from build123d import *

# Parameters (mm, degrees)
EXTRUDE_1_DEPTH     = 51.5
FILLET_2_R          = 6
SKETCH_2_W          = 41
SKETCH_2_H          = 41
CUT_EXTRUDE_1_DEPTH = 48.5
SKETCH_3_W          = 36
SKETCH_3_H          = 45.5
CUT_EXTRUDE_2_DEPTH = 54
SKETCH_4_W          = 36
SKETCH_4_H          = 45.5
CUT_EXTRUDE_3_DEPTH = 54
CUT_EXTRUDE_4_DEPTH = 6.5
CUT_EXTRUDE_5_DEPTH = 4


with BuildPart() as part:
    # 草图1 → 凸台-拉伸1 (new body)
    with BuildSketch(Plane(origin=(0, 0, 0), x_dir=(1, 0, 0), z_dir=(0, 1, 0))):
        with BuildLine():
            Line((-18, -24), (18, -24))
            ThreePointArc((18, -24), (22.242640687, -22.242640687), (24, -18))
            Line((24, -18), (24, 18))
            ThreePointArc((24, 18), (22.242640687, 22.242640687), (18, 24))
            Line((18, 24), (-18, 24))
            ThreePointArc((-18, 24), (-22.242640687, 22.242640687), (-24, 18))
            Line((-24, 18), (-24, -18))
            ThreePointArc((-24, -18), (-22.242640687, -22.242640687), (-18, -24))
        make_face()
    extrude(amount=EXTRUDE_1_DEPTH)

    # 圆角2
    fillet_2_edges = [part.edges().sort_by_distance(p)[0] for p in [
        (22.242640687, 51.5, -22.242640687),
        (24, 51.5, 0),
        (22.242640687, 51.5, 22.242640687),
        (0, 51.5, 24),
        (-22.242640687, 51.5, 22.242640687),
        (-24, 51.5, 0),
        (-22.242640687, 51.5, -22.242640687),
        (0, 51.5, -24),
    ]]
    fillet(fillet_2_edges, radius=FILLET_2_R)

    # 草图2 → 切除-拉伸1 (cut)
    with BuildSketch(Plane.XZ):
        Rectangle(SKETCH_2_W, SKETCH_2_H)
    extrude(amount=-CUT_EXTRUDE_1_DEPTH, mode=Mode.SUBTRACT)

    # 草图3 → 切除-拉伸2 (cut)
    with BuildSketch(Plane(origin=(0, 0, -24), x_dir=(-1, 0, 0), z_dir=(0, 0, -1))):
        with Locations((0, 22.75)):
            Rectangle(SKETCH_3_W, SKETCH_3_H)
    extrude(amount=-CUT_EXTRUDE_2_DEPTH, mode=Mode.SUBTRACT)

    # 草图4 → 切除-拉伸3 (cut)
    with BuildSketch(Plane.ZY.offset(24)):
        with Locations((0, 22.75)):
            Rectangle(SKETCH_4_W, SKETCH_4_H)
    extrude(amount=-CUT_EXTRUDE_3_DEPTH, mode=Mode.SUBTRACT)

    # 草图5 → 切除-拉伸4 (cut)
    with BuildSketch(Plane.XZ):
        with BuildLine():
            Line((-17.5, -23), (17.5, -23))
            ThreePointArc((17.5, -23), (21.389087297, -21.389087297), (23, -17.5))
            Line((23, -17.5), (23, 17.5))
            ThreePointArc((23, 17.5), (21.389087297, 21.389087297), (17.5, 23))
            Line((17.5, 23), (-17.5, 23))
            ThreePointArc((-17.5, 23), (-21.389087297, 21.389087297), (-23, 17.5))
            Line((-23, 17.5), (-23, -17.5))
            ThreePointArc((-23, -17.5), (-21.389087297, -21.389087297), (-17.5, -23))
        make_face()
    extrude(amount=-CUT_EXTRUDE_4_DEPTH, mode=Mode.SUBTRACT)

    # 草图8 → 切除-拉伸5 (cut)
    with BuildSketch(Plane.XZ):
        with BuildLine():
            Line((18, -22.977225575), (18, -24))
            ThreePointArc((18, -24), (22.242640687, -22.242640687), (24, -18))
            Line((24, -18), (22.977225575, -18))
            ThreePointArc((22.977225575, -18), (21.389087297, -21.389087297), (18, -22.977225575))
        make_face()
        with BuildLine():
            Line((22.977225575, 18), (24, 18))
            ThreePointArc((24, 18), (22.242640687, 22.242640687), (18, 24))
            Line((18, 24), (18, 22.977225575))
            ThreePointArc((18, 22.977225575), (21.389087297, 21.389087297), (22.977225575, 18))
        make_face()
        with BuildLine():
            Line((-18, 22.977225575), (-18, 24))
            ThreePointArc((-18, 24), (-22.242640687, 22.242640687), (-24, 18))
            Line((-24, 18), (-22.977225575, 18))
            ThreePointArc((-22.977225575, 18), (-21.389087297, 21.389087297), (-18, 22.977225575))
        make_face()
        with BuildLine():
            Line((-22.977225575, -18), (-24, -18))
            ThreePointArc((-24, -18), (-22.242640687, -22.242640687), (-18, -24))
            Line((-18, -24), (-18, -22.977225575))
            ThreePointArc((-18, -22.977225575), (-21.389087297, -21.389087297), (-22.977225575, -18))
        make_face()
    extrude(amount=-CUT_EXTRUDE_5_DEPTH, mode=Mode.SUBTRACT)


solid = part.part
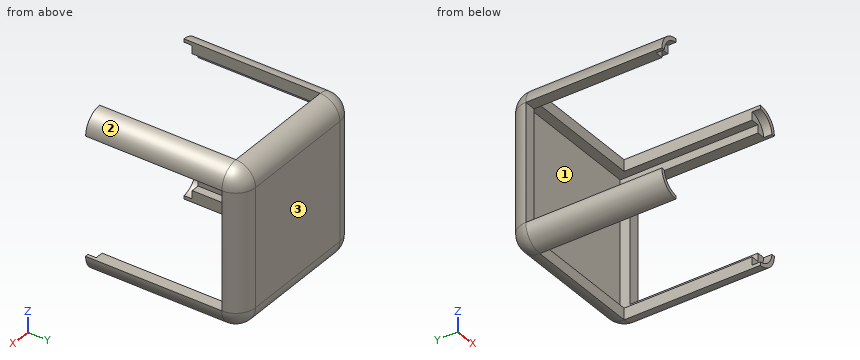
The listing builds one solid part. Answer for the finished solid, in the listing's coordinates (mm). Face numbers are marked on the shaded views. Give positions to 0.01 mm unless a question says otherwise; leave off trailing zeros. Loops run counter-clockwise (first coordinate to the right, second up) from the corner with the lowest first, then second, coordinate; pieces in that order, holes last. Notation, with made-up numbers: (32.25, 78.5) - (64.25, 78.5) arc R21 ccw to (64.25, 87.5) - close; hole circle Ø5 at (-40, 77.5). An arc over 180 degrees is marked (long way). Use one line per item in the form item = value.
1. Section D-D on x = -19 is taken. Give the vertices of the cut face in (y, z), then the cut area to 3 significant figures.
Calculated:
outline = (4, -23.92) - (45.5, -23.92) arc R5.92 ccw to (51.42, -18) - (51.42, 18) arc R5.92 ccw to (45.5, 23.92) - (4, 23.92) - (4, 22.79) - (6.5, 22.79) - (6.5, 20.5) - (48.5, 20.5) - (48.5, -20.5) - (6.5, -20.5) - (6.5, -22.79) - (4, -22.79) - close
area = 417 mm^2
2. Section B-B on x = 1 is taken. Give the vertices of the cut face in (y, z), then the cut area to 3 significant figures.
Calculated:
outline = (45.5, -24) arc R6 ccw to (51.5, -18) - (51.5, 18) arc R6 ccw to (45.5, 24) - (45.5, 20.5) - (48.5, 20.5) - (48.5, -20.5) - (45.5, -20.5) - close
area = 150 mm^2
3. Find the intervals of material crossed by line 1 along Y through (x, z) = (-7.5, 15); line 2 along X through (y, z) = (20.5, 19.5); line 3 along X through (y, z) = (42, -21.5), in increasing order. Write a range as [from, to].
Calculated:
line_1 = [48.5, 51.5]
line_2 = [-23.81, -20.5], [20.5, 23.81]
line_3 = [-22.87, -18], [18, 22.87]
4. Given pin 1 Ø4 at (x, y) = (-22, 25) entering from +Z; pin 2 Ø10 at (x, z) = (-3, 11.5) entering from -Y; pin 3 Ø3 at (x, z) = (21.5, 3.5) entering from -Y; pin 4 Ø20.5 at (y, z) = (34, 8) entering from +X, each flat-ended and moving along its own axis, determine where each tip first touches the part or whether it passes through.
Calculated:
pin_1 = 23.66
pin_2 = 48.5
pin_3 = 45.5
pin_4 = 24
5. Section A-A on y = 32.5 is taken. Give the vertices of the cut face in (x, z), then the cut area to 3 significant figures.
Calculated:
outline = (-24, -18) arc R6 ccw to (-18, -24) - (-18, -20.5) - (-20.5, -20.5) - (-20.5, -18) - close; (-24, 18) - (-20.5, 18) - (-20.5, 20.5) - (-18, 20.5) - (-18, 24) arc R6 ccw to start; (18, -24) arc R6 ccw to (24, -18) - (20.5, -18) - (20.5, -20.5) - (18, -20.5) - close; (18, 20.5) - (20.5, 20.5) - (20.5, 18) - (24, 18) arc R6 ccw to (18, 24) - close
area = 88.1 mm^2
6. Section C-C on z = -7 is taken. Give the vertices of the cut face in (x, y), then the cut area to 3 significant figures.
Calculated:
outline = (-24, 45.5) - (-20.5, 45.5) - (-20.5, 48.5) - (20.5, 48.5) - (20.5, 45.5) - (24, 45.5) arc R6 ccw to (18, 51.5) - (-18, 51.5) arc R6 ccw to start
area = 150 mm^2
7. The mould has two halves that part along Z. Classify the marked faces 1, 2 and 3: pulls with the +Z half, pulls with the -Z half, needs draft (parallel to the pull), parting line crosses it, or undercut.
Calculated:
face_1 = undercut
face_2 = pulls with the +Z half
face_3 = needs draft
